Study the drawing (mm; zero at the part's minimum x, y, z) and answer. Give positions to 0.01 mm unless a question says otherwise; leave off trailing zeros. Loops run counter-clockwise (first coordinate to the right, second up) from the corner with the lowest first, then second, coordinate; pieces in that order, holes last. Notation, with made-up numbers: M 78,72.25 L 96,72.25 A20 ccw 96,107.25 Z; hole C 57.25,-26 d2. An arc over 180 degrees is marked long. Return JSON: item names as keys, results as strings.
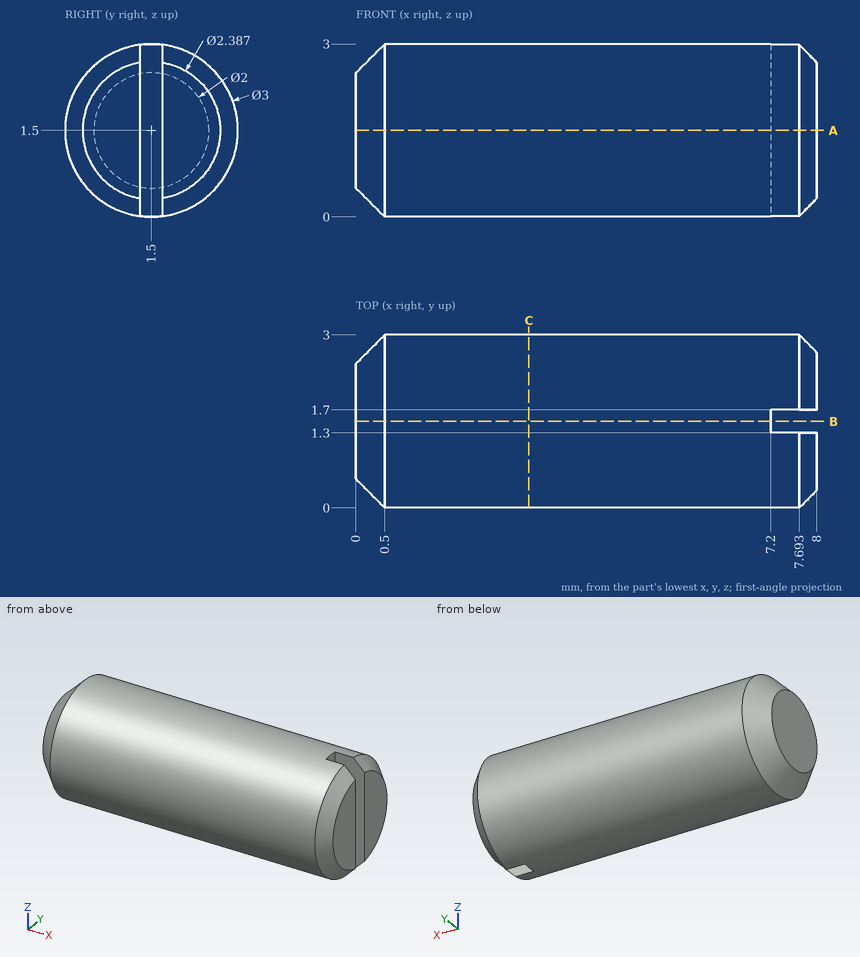
(1) Straight lines are drawn through the part: line 1 along X through (y, z) = (1.35, 2.35); line 2 along Y through (x, z) = (4.25, 1.3). For each, find the intervals that lie inside material, in ascending order.
Values follow:
{"line 1": "0 to 7.2", "line 2": "0.01 to 2.99"}
(2) The part is cut by section B-B (y = 1.5). Determine the outline of the cut face in (x, z).
Values follow:
{"outline": "M 0,0.5 L 0.5,0 L 7.2,0 L 7.2,3 L 0.5,3 L 0,2.5 Z"}
(3) Given pin 1 (1 mm diameter, centred on x = 5.5, z = 2, fed in from +Y), flat-ended and moving along its own axis, determine where the tip first touches the part or whether it passes through.
Values follow:
{"pin 1": "y = 3"}
(4) The part is cut by section A-A (z = 1.5). Determine the outline of the cut face in (x, y).
Values follow:
{"outline": "M 0,0.5 L 0.5,0 L 7.69,0 L 8,0.31 L 8,1.3 L 7.2,1.3 L 7.2,1.7 L 8,1.7 L 8,2.69 L 7.69,3 L 0.5,3 L 0,2.5 Z"}
(5) The part is cut by section C-C (x = 3). Determine the outline of the cut face in (y, z).
Values follow:
{"outline": "C 1.5,1.5 d3"}
